```python
from build123d import *

# Parameters (mm, degrees)
SKETCH2_R           = 7
SKETCH2_R_2         = 5
BOSS_EXTRUDE1_DEPTH = 4


with BuildPart() as part:
    # Sketch2 → Boss-Extrude1 (new body)
    with BuildSketch(Plane(origin=(0, 0, 0), x_dir=(0, 0, -1), z_dir=(1, 0, 0))):
        with BuildLine():
            Line((-77.539483891, 10.986864981), (204.077859883, 10.986864981))
            ThreePointArc((204.077859883, 10.986864981), (215.064724865, 0), (204.077859883, -10.986864981))
            Line((204.077859883, -10.986864981), (-77.539483891, -10.986864981))
            ThreePointArc((-77.539483891, -10.986864981), (-88.526348873, 0), (-77.539483891, 10.986864981))
        make_face()
        with Locations((-77.539483891, 0)):
            Circle(SKETCH2_R, mode=Mode.SUBTRACT)
        with Locations((204.077859883, 0)):
            Circle(SKETCH2_R, mode=Mode.SUBTRACT)
        with Locations((129.598441876, 0)):
            Circle(SKETCH2_R_2, mode=Mode.SUBTRACT)
    extrude(amount=BOSS_EXTRUDE1_DEPTH)


solid = part.part
```
Check sheet for the modelled part. Datum: model origin and axes. Units: mm. Coordinates: 2 decimals unless noted, no trailing zeros. Loops run counter-clockwise (first coordinate to the right, second up) from the corner with the lowest first, then second, coordinate; pieces in that order, holes last.
1) Gauge pin test, flat end, axial feed: pin 1 (11 mm diameter, centred on y = 0, z = 77.54, fed in from +X). Record the tip position at first contact, or that the pin passes through.
2) Sectioned sample at B-B (x = 1.2). Record the boundary of the cut face in (y, z), and give its area (3 significant figures).
3) Sectioned sample at A-A (y = 0). Record the boundary of the cut face in (x, z).
4) Release check for a two-part mould opening along Y. For faces 1 (the face through (4, 0, -65)), 2 (the face through (1.972, 0.22, -124.603)), 3 (the face through (1.972, -0.242, 88.524)) record: released by +Y, released by -Y, zero draft, split by the parting line, or undercut.
5) Material ranges on probe 1 along Z at (x, y) = (2.9, -0.5); probe 2 along Z at (x, y) = (0.2, 8.5); probe 3 along Z at (x, y) = (2.65, 5.5), recorded low to high.
Check sheet entries:
1. pin 1: passes through
2. outline: (-10.99, -204.08) arc R10.99 ccw to (10.99, -204.08) - (10.99, 77.54) arc R10.99 ccw to (-10.99, 77.54) - close; hole circle Ø14 at (0, -204.08); hole circle Ø14 at (0, 77.54); hole circle Ø10 at (0, -129.6)
2. area: 6,180 mm2
3. outline: (0, -215.06) - (4, -215.06) - (4, -211.08) - (0, -211.08) - close; (0, -197.08) - (4, -197.08) - (4, -134.6) - (0, -134.6) - close; (0, -124.6) - (4, -124.6) - (4, 70.54) - (0, 70.54) - close; (0, 84.54) - (4, 84.54) - (4, 88.53) - (0, 88.53) - close
4. face 1: zero draft
4. face 2: undercut
4. face 3: split by the parting line
5. probe 1: z = -215.05 to -211.06, -197.1 to -134.57, -124.62 to 70.56, 84.52 to 88.51
5. probe 2: z = -211.04 to 84.5
5. probe 3: z = -213.59 to -208.41, -199.75 to 73.21, 81.87 to 87.05
